For this review, take the finished solid that the model builds, in its own axes (mm). A direction names the side the tool comes from. Round coordinates to 2 decimals unless told otherwise and drop trailing zeros. Write each loop counter-clockwise with the first axis right and the second up, starting at its lowest first coordinate (ties: lowest second). Pieces come first, ordered by that corner, then holes. Notation, with made-up numbers: M 53.25,-35 L 92.25,-35 A25 ccw 92.25,-6 Z; hole C -30.5,-20.75 d8. An arc over 180 degrees is marked long. Answer in a Markdown table with one row per item.
```python
from build123d import *

# Parameters (mm, degrees)
SKETCH1_R               = 11
BOSS_EXTRUDE1_DEPTH     = 3
SKETCH2_R               = 4
BOSS_EXTRUDE2_DEPTH     = 14
SKETCH3_R               = 2
CUT_EXTRUDE1_DEPTH      = 20
BOSS_EXTRUDE3_START     = -3
BOSS_EXTRUDE3_OUTLINE_R = 1.75
BOSS_EXTRUDE3_DEPTH     = 3


# Read off the part's stored shape, not the designer's step: Boss-Extrude3
with BuildPart() as part:
    # Sketch1 → Boss-Extrude1 (new body)
    with BuildSketch(Plane(origin=(0, 0, 0), x_dir=(1, 0, 0), z_dir=(0, 1, 0))):
        with Locations(Location((0, 0, 0), (0, 0, 270))):
            Circle(SKETCH1_R)
    extrude(amount=BOSS_EXTRUDE1_DEPTH)

    # Sketch2 → Boss-Extrude2 (add)
    with BuildSketch(Plane(origin=(0, 3, 0), x_dir=(1, 0, 0), z_dir=(0, 1, 0))):
        with Locations(Location((0, 0, 0), (0, 0, 270))):
            Circle(SKETCH2_R)
    extrude(amount=BOSS_EXTRUDE2_DEPTH)

    # Sketch3 → Cut-Extrude1 (cut)
    with BuildSketch(Plane(origin=(0, 17, 0), x_dir=(1, 0, 0), z_dir=(0, 1, 0))):
        with Locations(Location((0, 0, 0), (0, 0, 270))):
            Circle(SKETCH3_R)
    extrude(amount=-CUT_EXTRUDE1_DEPTH, mode=Mode.SUBTRACT)

    # Boss-Extrude3 outline → Boss-Extrude3 (add)
    with BuildSketch(Plane.XZ.offset(BOSS_EXTRUDE3_START)):
        with BuildLine():
            ThreePointArc((-2.75, 14), (-4.710548646, 10.963037737), (-7.185731367, 8.328581195))
            ThreePointArc((-7.185731367, 8.328581195), (0, 11), (7.185731367, 8.328581195))
            ThreePointArc((7.185731367, 8.328581195), (4.710548646, 10.963037737), (2.75, 14))
            ThreePointArc((2.75, 14), (0, 16.75), (-2.75, 14))
        make_face()
        with Locations((0, 14)):
            Circle(BOSS_EXTRUDE3_OUTLINE_R, mode=Mode.SUBTRACT)
    extrude(amount=BOSS_EXTRUDE3_DEPTH)


solid = part.part
```
Q1. Take a section at A-A (z = 0). State the section outline as (x, y) points.
Found:
| item | result |
|---|---|
| outline | M -11,0 L -2,0 L -2,17 L -4,17 L -4,3 L -11,3 Z; M 2,0 L 11,0 L 11,3 L 4,3 L 4,17 L 2,17 Z |
Q2. For probe 1 along X at (y, z) = (4.75, 0); probe 2 along Y at (x, z) = (3, 11.5); probe 3 along Z at (x, y) = (7.25, 1), list the stretches that pass through material, from the lowest coordinate up.
Found:
| item | result |
|---|---|
| probe 1 | -4 to -2, 2 to 4 |
| probe 2 | 0 to 3 |
| probe 3 | -8.27 to 8.27 |
Q3. Take a section at D-D (z = 5.25). State the section outline as (x, y) points, then the cut area to 3 significant figures.
Found:
| item | result |
|---|---|
| outline | M -9.67,0 L 9.67,0 L 9.67,3 L -9.67,3 Z |
| area | 58.0 mm² |
Q4. Take a section at C-C (y = 15). State the section outline as (x, z) points.
Found:
| item | result |
|---|---|
| outline | C 0,0 d8; hole C 0,0 d4 |
Q5. Take a section at B-B (x = 0). State the section outline as (y, z) points.
Found:
| item | result |
|---|---|
| outline | M 0,-11 L 3,-11 L 3,-4 L 17,-4 L 17,-2 L 0,-2 Z; M 0,2 L 17,2 L 17,4 L 3,4 L 3,12.25 L 0,12.25 Z; M 0,15.75 L 3,15.75 L 3,16.75 L 0,16.75 Z |
Q6. Insertion check: P1, Ø1, axis at y = 12.5, z = 4, coming from the -X side; P2, Ø4.5, axis at x = 0, z = 14, coming from the +Y side; P3, Ø5, axis at y = 7, z = -5, coming from the -X side. Each pin has a flat end and moves straight along its axis. Give the tip position at first contact, or say it passes through.
Found:
| item | result |
|---|---|
| P1 | x = -1.94 |
| P2 | y = 3 |
| P3 | x = -3.12 |
Q7. Machinability: for faces 1 (the face through (-3, 3, 3)), 2 (the face through (0, 1, -11)), which of the approach directions +Z, -Z, +X, -X, +Y, -Y give a long, thin tool a straight path to every point of the face, cutting with its end or side? Answer none if there is none.
Found:
| item | result |
|---|---|
| face 1 | +Y |
| face 2 | +Y, -Y |
Q8. Mouldability with a two-part tool opening along X and no side actions: class faces 3 (the face through (4.742, 1.521, 10.923)), 4 (the face through (-3.905, 9.902, -0.867)), 5 (the face through (0, 0, 3)), 6 (the face through (-2, 9, 0)) as +X half, -X half, draft (parallel to the pull), parting line (faces both ways), or undercut.
Found:
| item | result |
|---|---|
| face 3 | +X half |
| face 4 | parting line |
| face 5 | draft |
| face 6 | undercut |
